```python
from build123d import *

# Parameters (mm, degrees)
PAD_DEPTH       = 8
THICKNESS_T     = -1.15
SKETCH002_R     = 1.6
PAD008_DEPTH    = 4
SKETCH011_W     = 15
SKETCH011_H     = 20
PAD009_DEPTH    = 10
SKETCH012_W     = 9.970298
SKETCH012_H     = 7.33189
POCKET002_DEPTH = 20
FILLET002_R     = 1
CHAMFER_SIZE    = 1
CHAMFER001_SIZE = 2


with BuildPart() as part:
    # Sketch001 → Pad (new body)
    with BuildSketch(Plane.XY):
        with BuildLine():
            Line((-25.25, 14), (-25.25, -14))
            ThreePointArc((-25.25, -14), (-24.298097, -16.298097), (-22, -17.25))
            Line((-22, -17.25), (22, -17.25))
            ThreePointArc((22, -17.25), (24.298097, -16.298097), (25.25, -14))
            Line((25.25, -14), (25.25, 14))
            ThreePointArc((25.25, 14), (24.298097, 16.298097), (22, 17.25))
            Line((22, 17.25), (-22, 17.25))
            ThreePointArc((-22, 17.25), (-24.298097, 16.298097), (-25.25, 14))
        make_face()
    extrude(amount=-PAD_DEPTH)

    # Thickness
    thickness_openings = [part.faces().sort_by_distance(p)[0] for p in [
        (0, 0, 0),
    ]]
    offset(amount=THICKNESS_T, openings=thickness_openings)

    # Sketch002 (on Face19 of Thickness) → Pad008 (join)
    with BuildSketch(Plane.XY.offset(-6.85)):
        with BuildLine():
            Line((-24.1, 14), (-24.1, 10.5))
            Line((-24.1, 10.5), (-21.5, 10.5))
            ThreePointArc((-21.5, 10.5), (-19.37868, 11.37868), (-18.5, 13.5))
            Line((-18.5, 13.5), (-18.5, 16.1))
            Line((-18.5, 16.1), (-22, 16.1))
            ThreePointArc((-22, 16.1), (-23.484924, 15.484924), (-24.1, 14))
        make_face()
        with Locations((-21.5, 13.5)):
            Circle(SKETCH002_R, mode=Mode.SUBTRACT)
        with BuildLine():
            Line((18.5, 16.1), (18.5, 13.5))
            ThreePointArc((18.5, 13.5), (19.37868, 11.37868), (21.5, 10.5))
            Line((21.5, 10.5), (24.1, 10.5))
            Line((24.1, 10.5), (24.1, 14))
            ThreePointArc((24.1, 14), (23.484924, 15.484924), (22, 16.1))
            Line((22, 16.1), (18.5, 16.1))
        make_face()
        with Locations((21.5, 13.5)):
            Circle(SKETCH002_R, mode=Mode.SUBTRACT)
        with BuildLine():
            Line((-21.5, -10.5), (-24.1, -10.5))
            Line((-24.1, -10.5), (-24.1, -14))
            ThreePointArc((-24.1, -14), (-23.484924, -15.484924), (-22, -16.1))
            Line((-22, -16.1), (-18.5, -16.1))
            Line((-18.5, -16.1), (-18.5, -13.5))
            ThreePointArc((-18.5, -13.5), (-19.37868, -11.37868), (-21.5, -10.5))
        make_face()
        with Locations((-21.5, -13.5)):
            Circle(SKETCH002_R, mode=Mode.SUBTRACT)
        with BuildLine():
            Line((18.5, -13.5), (18.5, -16.1))
            Line((18.5, -16.1), (22, -16.1))
            ThreePointArc((22, -16.1), (23.484924, -15.484924), (24.1, -14))
            Line((24.1, -14), (24.1, -10.5))
            Line((24.1, -10.5), (21.5, -10.5))
            ThreePointArc((21.5, -10.5), (19.37868, -11.37868), (18.5, -13.5))
        make_face()
        with Locations((21.5, -13.5)):
            Circle(SKETCH002_R, mode=Mode.SUBTRACT)
    extrude(amount=PAD008_DEPTH)

    # Sketch011 (on Face5 of Pad008) → Pad009 (join)
    with BuildSketch(Plane(origin=(0, 0, -8), x_dir=(1, 0, 0), z_dir=(0, 0, -1))):
        with Locations((-17, 0)):
            Rectangle(SKETCH011_W, SKETCH011_H)
    extrude(amount=PAD009_DEPTH)

    # Sketch012 (on Face19 of Pad009) → Pocket002 (cut)
    with BuildSketch(Plane(origin=(0, 10, 0), x_dir=(-1, 0, 0), z_dir=(0, 1, 0))):
        with Locations((14.327169, -11.723372)):
            Rectangle(SKETCH012_W, SKETCH012_H)
    extrude(amount=-POCKET002_DEPTH, mode=Mode.SUBTRACT)

    # Fillet002
    fillet002_edges = [part.edges().sort_by_distance(p)[0] for p in [
        (-19.312318, 0, -15.389317),
    ]]
    fillet(fillet002_edges, radius=FILLET002_R)

    # Chamfer
    chamfer_edges = [part.edges().sort_by_distance(p)[0] for p in [
        (-17, 10, -18),
        (-13.906159, 10, -15.389317),
        (-9.5, 0, -18),
        (-9.5, 0, -15.389317),
        (-13.906159, -10, -15.389317),
        (-17, -10, -18),
    ]]
    chamfer(chamfer_edges, length=CHAMFER_SIZE)

    # Chamfer001
    chamfer001_edges = [part.edges().sort_by_distance(p)[0] for p in [
        (-24.5, 0, -18),
    ]]
    chamfer(chamfer001_edges, length=CHAMFER001_SIZE)


solid = part.part
```
Geometry: final body of the model. Coordinates: model frame, mm. A direction names the side the tool comes from. Coordinates: 2 decimals unless noted, no trailing zeros. Loops run counter-clockwise (first coordinate to the right, second up) from the corner with the lowest first, then second, coordinate; pieces in that order, holes last. Notation, with made-up numbers: (52.25, 62.25) -> (69.25, 62.25) arc R28 cw to (69.25, 86.25) -> close; hole circle Ø4 at (-37, 38). An arc over 180 degrees is marked (long way). Use a Markdown table: item, result. Add a question column.
(1) Access query for faces 4 (the flat face through (-10, 0.1, -17.5)), 5 (the flat face through (-9.99, 0.14, -15.9)), 6 (the flat face through (21, -13, -6.85)). Directions: +Z, -Z, +X, -X, +Y, -Y. A direction counts if a zero-diameter tool reaches every point of the face in a straight line with its end or side. Return the directions, or none.
(2) Section query A-A, the plane z = -2.25. Return loops of the section in (x, y).
(3) Section query D-D, the plane y = 1. Return loops of the section in (x, z), plus the area to 3 significant figures.
(4) Mould query, pull axis Z, two halves, no side actions, for faces 1 (the flat face through (-20, -15, -2.85)), 2 (the flat face through (-13.84, -9.49, -15.88)), 3 (the flat face through (-23, 10.5, -5)). Classes: pulls with the +Z half, pulls with the -Z half, needs draft (parallel to the pull), parting line crosses it, or undercut.
(5) Line query: line 1 along Y through (x, z) = (21.5, -5.4); line 2 along Y through (x, z) = (-13, -3.75); line 3 along Z through (x, y) = (-11, 8.5). Output: solid intervals per line, ascending.
(6) Pin query (flat end, axial travel): pin 1 Ø3 at (x, z) = (-0.5, -10.5) entering from +Y; pin 2 Ø1.5 at (x, y) = (-11.5, 9.5) entering from +Z; pin 3 Ø3.5 at (x, y) = (21.5, -14) entering from +Z; pin 4 Ø4.5 at (x, z) = (-13.5, -13.5) entering from -Y. Return the tip coordinate at first contact, or that it passes through.
(7) Section query B-B, the plane x = 15.5. Return loops of the section in (y, z).
(8) Section query C-C, the plane z = -5.25. Return loops of the section in (x, y).
Answer:
| question | item | result |
|---|---|---|
| 1 | face 4 | -Z, +X, +Y, -Y |
| 1 | face 5 | +X, +Y, -Y |
| 1 | face 6 | +Z |
| 2 | outline | (-25.25, -14) arc R3.25 ccw to (-22, -17.25) -> (22, -17.25) arc R3.25 ccw to (25.25, -14) -> (25.25, 14) arc R3.25 ccw to (22, 17.25) -> (-22, 17.25) arc R3.25 ccw to (-25.25, 14) -> close; hole (-24.1, -14) arc R2.1 ccw to (-22, -16.1) -> (22, -16.1) arc R2.1 ccw to (24.1, -14) -> (24.1, 14) arc R2.1 ccw to (22, 16.1) -> (-22, 16.1) arc R2.1 ccw to (-24.1, 14) -> close |
| 3 | outline | (-25.25, -8) -> (-24.5, -8) -> (-24.5, -16) -> (-22.5, -18) -> (-10.5, -18) -> (-9.5, -17) -> (-9.5, -16.39) -> (-10.5, -15.39) -> (-18.31, -15.39) arc R1 cw to (-19.31, -14.39) -> (-19.31, -8.06) -> (-9.5, -8.06) -> (-9.5, -8) -> (25.25, -8) -> (25.25, 0) -> (24.1, 0) -> (24.1, -6.85) -> (-24.1, -6.85) -> (-24.1, 0) -> (-25.25, 0) -> close |
| 3 | area | 149 mm^2 |
| 4 | face 1 | pulls with the +Z half |
| 4 | face 2 | undercut |
| 4 | face 3 | needs draft |
| 5 | line 1 | y = -17.25 to -15.1, -11.9 to -10.5, 10.5 to 11.9, 15.1 to 17.25 |
| 5 | line 2 | y = -17.25 to -16.1, 16.1 to 17.25 |
| 5 | line 3 | z = -18 to -15.39, -8.06 to -6.85 |
| 6 | pin 1 | passes through |
| 6 | pin 2 | stops at z = -6.85 |
| 6 | pin 3 | stops at z = -2.85 |
| 6 | pin 4 | stops at y = -9.36 |
| 7 | outline | (-17.25, -8) -> (17.25, -8) -> (17.25, 0) -> (16.1, 0) -> (16.1, -6.85) -> (-16.1, -6.85) -> (-16.1, 0) -> (-17.25, 0) -> close |
| 8 | outline | (-25.25, -14) arc R3.25 ccw to (-22, -17.25) -> (22, -17.25) arc R3.25 ccw to (25.25, -14) -> (25.25, 14) arc R3.25 ccw to (22, 17.25) -> (-22, 17.25) arc R3.25 ccw to (-25.25, 14) -> close; hole (-24.1, -10.5) -> (-21.5, -10.5) arc R3 cw to (-18.5, -13.5) -> (-18.5, -16.1) -> (18.5, -16.1) -> (18.5, -13.5) arc R3 cw to (21.5, -10.5) -> (24.1, -10.5) -> (24.1, 10.5) -> (21.5, 10.5) arc R3 cw to (18.5, 13.5) -> (18.5, 16.1) -> (-18.5, 16.1) -> (-18.5, 13.5) arc R3 cw to (-21.5, 10.5) -> (-24.1, 10.5) -> close; hole circle Ø3.2 at (-21.5, -13.5); hole circle Ø3.2 at (-21.5, 13.5); hole circle Ø3.2 at (21.5, -13.5); hole circle Ø3.2 at (21.5, 13.5) |
